```python
from build123d import *

# Parameters (mm, degrees)
F0_W     = 74
F0_H     = 74
F1_DEPTH = 900
F2_W     = 74
F2_H     = 58
F4_DEPTH = 38
F3_W     = 74
F3_H     = 58
F5_DEPTH = 38
F7_D     = 12
F7_DEPTH = 40
F7_TIP   = 3.6051637142
F8_W     = 74
F8_H     = 58
F9_DEPTH = 38
F10_R    = 5


with BuildPart() as f1:
    # F0 (on Top) → F1 (new body)
    with BuildSketch(Plane.XY):
        Rectangle(F0_W, F0_H)
    extrude(amount=-F1_DEPTH)

    # F2 (on face) → F4 (cut)
    with BuildSketch(Plane.XZ.offset(37)):
        with Locations((0, -29)):
            Rectangle(F2_W, F2_H)
    extrude(amount=-F4_DEPTH, mode=Mode.SUBTRACT)

    # F3 (on face) → F5 (cut)
    with BuildSketch(Plane(origin=(-37, 0, 0), x_dir=(0, -1, 0), z_dir=(-1, 0, 0))):
        with Locations((0, -29)):
            Rectangle(F3_W, F3_H)
    extrude(amount=-F5_DEPTH, mode=Mode.SUBTRACT)

    # F7
    with Locations(Plane.XY.offset(-58)):
        with Locations((-18, -18)):
            Hole(F7_D / 2, depth=F7_DEPTH)
            with Locations((0, 0, -(F7_DEPTH + F7_TIP / 2))):  # 118° drill point
                Cone(0, F7_D / 2, F7_TIP, mode=Mode.SUBTRACT)

    # F8 (on face) → F9 (cut)
    with BuildSketch(Plane(origin=(-37, 0, 0), x_dir=(0, -1, 0), z_dir=(-1, 0, 0))):
        with Locations((0, -771)):
            Rectangle(F8_W, F8_H)
    extrude(amount=-F9_DEPTH, mode=Mode.SUBTRACT)

    # F10
    f10_edges = [f1.edges().sort_by_distance(p)[0] for p in [
        (-37, -37, -850),
        (-37, -37, -400),
        (-37, 37, -400),
        (-37, 37, -850),
        (37, -37, -479),
        (37, 37, -450),
    ]]
    fillet(f10_edges, radius=F10_R)


solid = f1.part
```
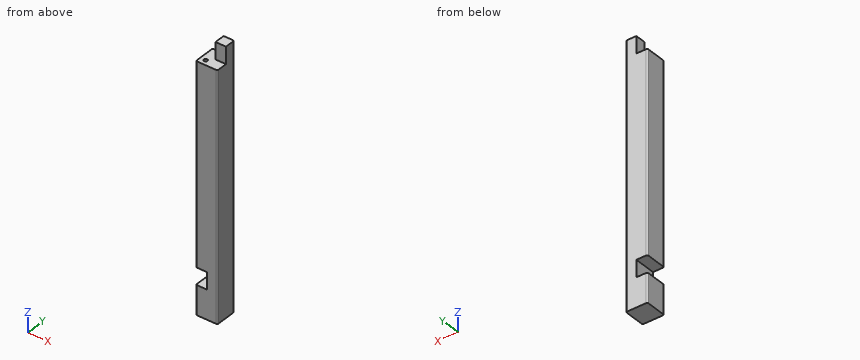
The model under review builds one solid part; all positions refer to its coordinate system, in mm. Round coordinates to 2 decimals unless told otherwise and drop trailing zeros. Loops run counter-clockwise (first coordinate to the right, second up) from the corner with the lowest first, then second, coordinate; pieces in that order, holes last. Notation, with made-up numbers: (-29, 66) - (1, 66) arc R23 ccw to (1, 76) - close; hole circle Ø9 at (67, 88.5). An arc over 180 degrees is marked (long way). Write each question's results on one line, items separated by ' | '. Start each with the question number.
Q1. Take a section at A-A on z = -752. Give the boundary of the cut face in (x, y).
Q2. Insertion check: P1, Ø11, axis at x = 16, z = -17.5, coming from the -Y side; P2, Ø12, axis at x = 10.5, y = -11, coming from the +Z side; P3, Ø17.5, axis at y = 15, z = -763, coming from the -X side. Each pin has a flat end and moves straight along its axis. Give the tip position at first contact, or say it passes through.
Q3. Wall thickness on line 1 along X through (y, z) = (-18, -72); line 2 along Z through (x, y) = (-23, -14.5): over which ranges is each line inside the solid? List them lowest first. Write a range as [from, to].
Q4. Take a section at C-C on x = 20. Give the boundary of the cut face in (y, z).
Q5. Take a section at B-B on y = 19.5. Give the boundary of the cut face in (x, z).
Data:
1) outline: (1, -37) - (32, -37) arc R5 ccw to (37, -32) - (37, 32) arc R5 ccw to (32, 37) - (1, 37) - close
2) P1: stops at y = 1 | P2: stops at z = -58 | P3: stops at x = 1
3) line 1: x = [-37, -24], [-12, 37] | line 2: z = [-900, -800], [-742, -58]
4) outline: (-37, -900) - (37, -900) - (37, 0) - (1, 0) - (1, -58) - (-37, -58) - close
5) outline: (-37, -900) - (37, -900) - (37, 0) - (1, 0) - (1, -58) - (-37, -58) - (-37, -742) - (1, -742) - (1, -800) - (-37, -800) - close
